Geometry check sheet. Reference: the model listing, model coordinates, mm. A direction names the side the tool comes from. Round coordinates to 2 decimals unless told otherwise and drop trailing zeros. Write each loop counter-clockwise with the first axis right and the second up, starting at its lowest first coordinate (ties: lowest second). Pieces come first, ordered by that corner, then holes. Notation, with made-up numbers: (79, 42) -> (87, 42) arc R23 ccw to (87, 75) -> close; hole circle Ø2 at (49.5, -26.5). An arc over 180 degrees is marked (long way). Put each result on its own line as item: value. Start each with the question number.
from build123d import *

# Parameters (mm, degrees)
F1_DEPTH      = 14
F2_R          = 8
F3_DEPTH      = 11
F4_R          = 3.5
F5_DEPTH      = 14.001
F5_DEPTH_BACK = 14.001
F6_R          = 2
F7_DEPTH      = 11.001
F8_R          = 11
F8_R_2        = 10
F9_DEPTH      = 1.5
F10_R         = 0.5


with BuildPart() as f1:
    # F0 (on Front) → F1 (new body, symmetric)
    with BuildSketch(Plane.XZ):
        with BuildLine():
            Line((8, 0), (11, 0))
            ThreePointArc((11, 0), (0, 11), (-11, 0))
            Line((-11, 0), (-8, 0))
            Line((-8, 0), (8, 0))
        make_face()
    extrude(amount=F1_DEPTH, both=True)

    # F2 (on Front) → F3 (cut, symmetric)
    with BuildSketch(Plane.XZ):
        Circle(F2_R)
    extrude(amount=F3_DEPTH, both=True, mode=Mode.SUBTRACT)

    # F4 (on Front) → F5 (cut, two sides)
    with BuildSketch(Plane.XZ) as f5_sk:
        Circle(F4_R)
    extrude(amount=-F5_DEPTH, mode=Mode.SUBTRACT)
    extrude(f5_sk.sketch, amount=F5_DEPTH_BACK, mode=Mode.SUBTRACT)

    # F6 (on Top) → F7 (cut, through all)
    with BuildSketch(Plane.XY):
        with Locations((4.8, 7.5)):
            Circle(F6_R)
        with Locations((-4.8, 7.5)):
            Circle(F6_R)
        with Locations((4.8, -7.5)):
            Circle(F6_R)
        with Locations((-4.8, -7.5)):
            Circle(F6_R)
    extrude(amount=F7_DEPTH, mode=Mode.SUBTRACT)

    # F8 (on Front) → F9 (cut, symmetric)
    with BuildSketch(Plane.XZ):
        Circle(F8_R)
        Circle(F8_R_2, mode=Mode.SUBTRACT)
    extrude(amount=F9_DEPTH, both=True, mode=Mode.SUBTRACT)

    # F10
    f10_edges = [f1.edges().sort_by_distance(p)[0] for p in [
        (0, 1.5, 10),
        (0, -1.5, 10),
        (0, 14, 11),
        (0, -14, 11),
        (0, 11, 8),
        (0, -11, 8),
    ]]
    fillet(f10_edges, radius=F10_R)


solid = f1.part
(1) Material ranges on L1, parallel to Y at x = 4.8, z = 7; L2, parallel to Y at x = -4, z = 9.75; L3, parallel to X at y = -7.5, z = 9.25, recorded low to high. Write a range as from..to.
(2) Sectioned sample at C-C (y = -7.5). Record the cut outline in (x, z), and give its area (3 significant figures).
(3) Sectioned sample at A-A (x = 0). Record the cut outline in (y, z), and give its area (3 significant figures).
(4) Set-up check for faces 4 (the cylindrical face through (0.1, -12.5, 3.5)), 5 (the flat face through (0, 11, 4)), 6 (the flat face through (-0.1, 1.5, 10.8)): record each of +Z, -Z, +X, -X, +Y, -Y from which the full face is reachable in a straight line by a thin tool's end or side.
(5) Go/stop test with flat-tipped pins: pin 1 Ø2 at (y, z) = (8, 7.5) entering from -X; pin 2 Ø6 at (x, y) = (7.5, 6.5) entering from +Z; pin 3 Ø5 at (x, y) = (4.8, -7.5) entering from +Z. Record where each tip stops, or that it passes through.
(6) Mould release check, pull along X, two halves, no side actions. Record for faces 1 (the cylindrical face through (0, 0, 8)), 2 (the cylindrical face through (0, -8, 11)), 3 (the flat face through (0, -14, 5)): +X half, -X half, draft (parallel to the pull), parting line (faces both ways), or undercut.
(7) Sectioned sample at D-D (x = 4.5). State how many separate pieces and enclosed holes the cut face has, and give its area (3 significant figures).
(8) Sectioned sample at B-B (y = 6.5). Record the cut outline in (x, z).
Found:
1. L1: -14..-9.5, -5.5..5.5, 9.5..14
1. L2: -14..-9.33, -5.67..-1.5, 1.5..5.67, 9.33..14
1. L3: -2.8..2.8
2. outline: (-11, 0) -> (-8, 0) arc R8 cw to (-6.8, 4.21) -> (-6.8, 8.65) arc R11 ccw to start; (-2.8, 7.49) arc R8 cw to (2.8, 7.49) -> (2.8, 10.64) arc R11 ccw to (-2.8, 10.64) -> close; (6.8, 4.21) arc R8 cw to (8, 0) -> (11, 0) arc R11 ccw to (6.8, 8.65) -> close
2. area: 60.8 mm2
3. outline: (-14, 3.5) -> (-11, 3.5) -> (-11, 7.5) arc R0.5 cw to (-10.5, 8) -> (10.5, 8) arc R0.5 cw to (11, 7.5) -> (11, 3.5) -> (14, 3.5) -> (14, 10.5) arc R0.5 ccw to (13.5, 11) -> (1.5, 11) -> (1.5, 10.5) arc R0.5 cw to (1, 10) -> (-1, 10) arc R0.5 cw to (-1.5, 10.5) -> (-1.5, 11) -> (-13.5, 11) arc R0.5 ccw to (-14, 10.5) -> close
3. area: 108 mm2
4. face 4: -Z, +Y, -Y
4. face 5: -Z
4. face 6: +Z
5. pin 1: x = -8.87
5. pin 2: z = 9.96
5. pin 3: z = 10.76
6. face 1: undercut
6. face 2: parting line
6. face 3: draft
7. separate pieces: 3
7. enclosed holes: 0
7. area: 105 mm2
8. outline: (-11, 0) -> (-8, 0) arc R8 cw to (-6.53, 4.62) -> (-6.53, 8.85) arc R11 ccw to start; (-3.07, 7.39) arc R8 cw to (3.07, 7.39) -> (3.07, 10.56) arc R11 ccw to (-3.07, 10.56) -> close; (6.53, 4.62) arc R8 cw to (8, 0) -> (11, 0) arc R11 ccw to (6.53, 8.85) -> close
